Autodesk Inventor part; units mm, degrees
ref_plane "YZ Plane" through (0, 0, 0) normal (1, 0, 0) x (0, 1, 0)
ref_plane "XZ Plane" through (0, 0, 0) normal (0, 1, 0) x (-1, 0, 0)
ref_plane "XY Plane" through (0, 0, 0) normal (0, 0, 1) x (1, 0, 0)
sketch "Boceto1" plane through (0, 0, 0) normal (0, 1, 0) x (-1, 0, 0)
  line L0 (0, 0) -> (30, 0)
  line L1 (30, 0) -> (30, -60)
  line L2 (30, -60) -> (0, -60)
  line L3 (0, -60) -> (0, 0)
  dimension "d0" = 60
  dimension "d1" = 30
extrude "Extrusión1" add sketch "Boceto1" along normal blind 1000
sketch "Boceto2" plane through (0, 0, 0) normal (0, -1, 0) x (1, 0, 0)
  line L0 (-1.2, -1.2) -> (-28.8, -1.2)
  line L1 (-28.8, -1.2) -> (-28.8, -58.8)
  line L2 (-28.8, -58.8) -> (-1.2, -58.8)
  line L3 (-1.2, -58.8) -> (-1.2, -1.2)
  line L4 (0, 0) -> (0, -60)
  line L5 (-30, -60) -> (-30, 0)
  line L6 (-30, 0) -> (0, 0)
  line L7 (0, -60) -> (-30, -60)
  dimension "d4" = 1.2
  dimension "d5" = 1.2
  dimension "d6" = 1.2
  dimension "d7" = 1.2
extrude "Extrusión2" cut sketch "Boceto2" against normal through all contours L3 L2 L1 L0
sketch "Boceto3" plane through (-30, 0, 0) normal (0, 0, 1) x (1, 0, 0)
  line L0 (30, 0) -> (1.2, 0)
  line L1 (1.2, 0) -> (1.2, 66)
  line L2 (1.2, 66) -> (30, 66)
  line L3 (30, 66) -> (30, 0)
  line L4 (0, 0) -> (0, 1000)
  dimension "d10" = 1.2
  dimension "d11" = 66
extrude "Extrusión3" cut sketch "Boceto3" against normal through all
sketch "Boceto4" plane through (-28.8, 0, 0) normal (1, 0, 0) x (0, 0, -1)
  point P0 (0, 0)
sketch "Boceto5" plane through (-30, 0, -60) normal (-1, 0, 0) x (0, 0, 1)
  line L0 (60, 0) -> (0, 0)
  line L1 (0, 0) -> (0, -2)
  line L2 (0, -2) -> (60, -2)
  line L3 (60, -2) -> (60, 0)
  dimension "d14" = 2
extrude "Extrusión4" add sketch "Boceto5" against normal blind 30
properties part number "Expendedor"
Geometry: final body of the model. Coordinates: model frame, mm. A direction names the side the tool comes from. Coordinates: 2 decimals unless noted, no trailing zeros. Loops run counter-clockwise (first coordinate to the right, second up) from the corner with the lowest first, then second, coordinate; pieces in that order, holes last. Notation, with made-up numbers: (52.25, -27) -> (86.25, -27) arc R32 cw to (86.25, 4) -> close; hole circle Ø7 at (-19, 28). An arc over 180 degrees is marked (long way). Use a Markdown table: item, result. Add a question column.
(1) Pin query (flat end, axial travel): pin 1 Ø14.5 at (x, z) = (-12.5, -19) entering from +Y; pin 2 Ø6 at (y, z) = (888.5, -43.5) entering from +X. Return the tip coordinate at first contact, or that it passes through.
(2) Mould query, pull axis X, two halves, no side actions, for faces 1 (the flat face through (-15, 617, -60)), 2 (the flat face through (-1.2, 526, -30)), 3 (the flat face through (-28.8, 493, -30)), 4 (the flat face through (-30, 506, -30)). Classes: pulls with the +X half, pulls with the -X half, needs draft (parallel to the pull), parting line crosses it, or undercut.
(3) Access query for faces 5 (the flat face through (-15, 492, 0)), 6 (the flat face through (-15, 526, -58.8)), 7 (the flat face through (-1, 66, -17)). Directions: +Z, -Z, +X, -X, +Y, -Y. A direction counts if a zero-diameter tool reaches every point of the face in a straight line with its end or side. Return the directions, or none.
(4) Line query: line 1 along X through (y, z) = (845.5, -20.5); line 2 along Z through (x, y) = (-27.25, 449); line 3 along Y through (x, z) = (-20.5, -26.5). Output: solid intervals per line, ascending.
(5) Section query C-C, the plane y = 782. Return loops of the section in (x, z), plus the area to 3 significant figures.
(6) Section query A-A, the plane z = -17.5. Return loops of the section in (x, y).
(7) Section query B-B, the plane x = -16.25. Return loops of the section in (y, z), plus the area to 3 significant figures.
Answer:
| question | item | result |
|---|---|---|
| 1 | pin 1 | stops at y = 0 |
| 1 | pin 2 | stops at x = 0 |
| 2 | face 1 | needs draft |
| 2 | face 2 | undercut |
| 2 | face 3 | undercut |
| 2 | face 4 | pulls with the -X half |
| 3 | face 5 | +Z, +X, -X, +Y, -Y |
| 3 | face 6 | +Y |
| 3 | face 7 | +Z, -Z, +X |
| 4 | line 1 | x = -30 to -28.8, -1.2 to 0 |
| 4 | line 2 | z = -60 to -58.8, -1.2 to 0 |
| 4 | line 3 | y = -2 to 0 |
| 5 | outline | (-30, -60) -> (0, -60) -> (0, 0) -> (-30, 0) -> close; hole (-28.8, -58.8) -> (-1.2, -58.8) -> (-1.2, -1.2) -> (-28.8, -1.2) -> close |
| 5 | area | 210 mm^2 |
| 6 | outline | (-30, -2) -> (0, -2) -> (0, 0) -> (-28.8, 0) -> (-28.8, 1000) -> (-30, 1000) -> close; (-1.2, 66) -> (0, 66) -> (0, 1000) -> (-1.2, 1000) -> close |
| 7 | outline | (-2, -60) -> (0, -60) -> (0, 0) -> (-2, 0) -> close; (66, -60) -> (1000, -60) -> (1000, -58.8) -> (66, -58.8) -> close; (66, -1.2) -> (1000, -1.2) -> (1000, 0) -> (66, 0) -> close |
| 7 | area | 2,360 mm^2 |
